Build history of the part. All positions in model axes, mm. A direction names the side the tool comes from. Round coordinates to 2 decimals unless told otherwise and drop trailing zeros. Write each loop counter-clockwise with the first axis right and the second up, starting at its lowest first coordinate (ties: lowest second). Pieces come first, ordered by that corner, then holes. Notation, with made-up numbers: M -11.75,-20.5 L 14.25,-20.5 A9 cw 14.25,-13.5 Z; hole C 36.25,50.5 d9. An arc over 180 degrees is marked long. Write item = value, one per line. Start each with the question number.
Q1. Band-saw the part on D-D on x = -5. Write the cut outline in (y, z), plus the area to 3 significant figures.
Q2. Band-saw the part on B-B on y = 12. Write the cut outline in (x, z) (3 decimals), plus the area to 3 significant figures.
Q3. Probe L1, parallel to X at y = 2.6, z = 0; L2, parallel to Z at x = 0, y = 10.5 (3 decimals); L3, parallel to Y at x = -0.25, z = 0.5. List the from-to ranges inside material, lowest first.
Q4. Pull direction X, two halves, no side cores. Call faces 4 (the flat face through (2.6, 8, 7.2)), 5 (the cylindrical face through (-10.74, 3.94, -2.38)), 6 (the conical face through (0.12, 6.745, 8.231)): released by +X, released by -X, zero draft, split by the parting line, or undercut.
Q5. Band-saw the part on A-A on y = 4. Write the cut outline in (x, z).
Q6. Tool access for faces 1 (the cylindrical face through (-9.464, 3.203, -0.325)), 2 (the cylindrical face through (-0.071, 10.877, -5.937)), 3 (the cylindrical face through (-2.87, 11.94, 6.93)): list every direction of +Z, -Z, +X, -X, +Y, -Y with a clear straight run to the whole face (end or side of a thin tool).
Q7. Band-saw the part on C-C on z = -5.5. Write the cut outline in (x, y) (3 decimals), plus the area to 3 significant figures.
Q8. Drop flat-ended pins along their axis: P1, Ø1, axis at x = 7.5, y = 3, coming from the +Z side; P2, Ø7.5, axis at x = 0, z = 0, coming from the +Y side; P3, Ø8, axis at x = -2.5, y = 11.5, coming from the +Z side. Give the stop position or say it passes through.
```python
from build123d import *

# Parameters (mm, degrees)
SKETCH1_R           = 11
BOSS_EXTRUDE1_DEPTH = 8
SKETCH2_R           = 7.5
BOSS_EXTRUDE2_DEPTH = 8
SKETCH3_R           = 4.625
CUT_EXTRUDE1_DEPTH  = 8
CIRPATTERN1_COUNT   = 4
SKETCH10_W          = 1.625
SKETCH10_H          = 11


with BuildPart() as part:
    # Sketch1 → Boss-Extrude1 (new body)
    with BuildSketch(Plane(origin=(0, 0, 0), x_dir=(1, 0, 0), z_dir=(0, 1, 0))):
        with Locations(Location((0, 0, 0), (0, 0, 270))):
            Circle(SKETCH1_R)
    extrude(amount=BOSS_EXTRUDE1_DEPTH)

    # Sketch2 → Boss-Extrude2 (add)
    with BuildSketch(Plane(origin=(0, 8, 0), x_dir=(1, 0, 0), z_dir=(0, 1, 0))):
        with Locations(Location((0, 0, 0), (0, 0, 270))):
            Circle(SKETCH2_R)
    extrude(amount=BOSS_EXTRUDE2_DEPTH)

    # Sketch3 → Cut-Extrude1 (cut)
    with BuildSketch(Plane(origin=(0, 16, 0), x_dir=(1, 0, 0), z_dir=(0, 1, 0))):
        with Locations(Location((0, 0, 0), (0, 0, 270))):
            Circle(SKETCH3_R)
    extrude(amount=-CUT_EXTRUDE1_DEPTH, mode=Mode.SUBTRACT)

    # Sketch7 → Ø3.0mm Dowel Hole1 (revolve, cut)
    with BuildSketch(Plane(origin=(8, 0, 0), x_dir=(0, 0, -1), z_dir=(1, 0, 0))):
        Polygon((0, 0), (0, 6.901290929), (1.5, 6), (1.5, 0.482842712), (1.7, 0), align=None)
    f_3_0mm_dowel_hole1 = revolve(axis=Axis((8, -6.35, 0), (0, 1, 0)), mode=Mode.SUBTRACT)

    # CirPattern1: Ø3.0mm Dowel Hole1 ×4 about axis
    cirpattern1_axis = Axis((0, 0, 0), (0, 1, 0))
    for i in range(1, CIRPATTERN1_COUNT):
        add(f_3_0mm_dowel_hole1.rotate(cirpattern1_axis, i * 360 / CIRPATTERN1_COUNT), mode=Mode.SUBTRACT)

    # Sketch10 → Ø5.0mm Dowel Hole1 (revolve, cut)
    with BuildSketch(Plane(origin=(0, 12.5, 0), x_dir=(0, 1, 0), z_dir=(1, 0, 0))):
        with Locations((0.8125, 5.5)):
            Rectangle(SKETCH10_W, SKETCH10_H)
    f_5_0mm_dowel_hole1 = revolve(axis=Axis((0, 12.5, -6.35), (0, 0, 1)), mode=Mode.SUBTRACT)

    # Mirror1: Ø5.0mm Dowel Hole1 across plane
    add(f_5_0mm_dowel_hole1.mirror(Plane.XY), mode=Mode.SUBTRACT)


solid = part.part
```
Conclusion:
q1.outline = M 0,-9.8 L 8,-9.8 L 8,-5.59 L 16,-5.59 L 16,5.59 L 8,5.59 L 8,9.8 L 0,9.8 Z
q1.area = 246 mm^2
q2.outline = M -1.546,-7.339 L -1.546,-4.359 A4.625 cw -1.546,4.359 L -1.546,7.339 A7.5 ccw Z; M 1.546,-7.339 A7.5 ccw 1.546,7.339 L 1.546,4.359 A4.625 cw 1.546,-4.359 Z
q2.area = 91.5 mm^2
q3.L1 = -11 to -9.5, -6.5 to 6.5, 9.5 to 11
q3.L2 = -7.5 to -4.625, 4.625 to 7.5
q3.L3 = 0 to 8
q4.face_4 = zero draft
q4.face_5 = split by the parting line
q4.face_6 = undercut
q5.outline = C 0,0 d22; hole C -8,0 d3; hole C 0,-8 d3; hole C 0,8 d3; hole C 8,0 d3
q6.face_1 = -Y
q6.face_2 = +Z, -Z
q6.face_3 = +Y
q7.outline = M -9.526,0 L 9.526,0 L 9.526,8 L 5.099,8 L 5.099,16 L -5.099,16 L -5.099,8 L -9.526,8 Z; hole C 0,12.5 d3.25
q7.area = 226 mm^2
q8.P1 = 8.49
q8.P2 = 8
q8.P3 = 10.99
